Input: part model. Units: mm. Frame: model coordinates. A direction names the side the tool comes from. Round coordinates to 2 decimals unless told otherwise and drop trailing zeros. Order: outer loops, then holes, each group sorted by start corner. A loop starts at its lowest first (then second) coordinate and runs counter-clockwise, first axis right, second up. Notation, with made-up numbers: M 30.25,28 L 68.25,28 A16 ccw 68.25,55 Z; hole C 38,49.25 d7. An arc over 180 degrees is marked long. One line per question, with ' | ' between items.
```python
from build123d import *

# Parameters (mm, degrees)
SALIENTE_EXTRUIR1_DEPTH = 20
CROQUIS2_R              = 20
SALIENTE_EXTRUIR2_DEPTH = 35
CORTAR_EXTRUIR1_DEPTH   = 15
CORTAR_EXTRUIR2_REACH   = 68.332
CROQUIS4_R              = 4
CROQUIS5_R              = 12.5
CROQUIS5_R_2            = 6
SALIENTE_EXTRUIR3_DEPTH = 48
REDONDEO1_R             = 3
NERVIO1_REACH           = 91.22
CROQUIS6_WALL_W         = 207.940466532
CROQUIS6_WALL_H         = 6


with BuildPart() as part:
    # Croquis1 → Saliente-Extruir1 (new body)
    with BuildSketch(Plane.XY):
        with BuildLine():
            Line((-12.5, -26.339134382), (-12.5, -60))
            ThreePointArc((-12.5, -60), (0, -47.5), (12.5, -60))
            Line((12.5, -60), (12.5, -26.339134382))
            ThreePointArc((12.5, -26.339134382), (13.646923907, -18.12329602), (17, -10.535653753))
            ThreePointArc((17, -10.535653753), (0, -20), (-17, -10.535653753))
            ThreePointArc((-17, -10.535653753), (-13.646923907, -18.12329602), (-12.5, -26.339134382))
        make_face()
    extrude(amount=SALIENTE_EXTRUIR1_DEPTH)

    # Croquis2 → Saliente-Extruir2 (add)
    with BuildSketch(Plane.XY):
        with Locations(Location((0, 0, 0), (0, 0, 211.788330617))):
            Circle(CROQUIS2_R)
    extrude(amount=SALIENTE_EXTRUIR2_DEPTH)

    # Croquis3 → Cortar-Extruir1 (cut)
    with BuildSketch(Plane.XY.offset(35)):
        with BuildLine():
            Line((-3, 11.618950039), (-3, 8))
            Line((-3, 8), (3, 8))
            Line((3, 8), (3, 11.618950039))
            ThreePointArc((3, 11.618950039), (12, 0), (3, -11.618950039))
            Line((3, -11.618950039), (3, -8))
            Line((3, -8), (-3, -8))
            Line((-3, -8), (-3, -11.618950039))
            ThreePointArc((-3, -11.618950039), (-12, 0), (-3, 11.618950039))
        make_face()
    extrude(amount=-CORTAR_EXTRUIR1_DEPTH, mode=Mode.SUBTRACT)

    # Croquis4 → Cortar-Extruir2 (cut, up to next)
    with BuildSketch(Plane.XY.offset(20), mode=Mode.PRIVATE) as cortar_extruir2_sk1:
        Circle(CROQUIS4_R)
    cortar_extruir2_tool1 = extrude(cortar_extruir2_sk1.sketch, amount=-CORTAR_EXTRUIR2_REACH, mode=Mode.PRIVATE) & part.part
    add(cortar_extruir2_tool1.solids().sort_by_distance((0, 0, 20))[0], mode=Mode.SUBTRACT)

    # Croquis5 → Saliente-Extruir3 (add)
    with BuildSketch(Plane.XY):
        with Locations((0, -60)):
            Circle(CROQUIS5_R)
        with Locations((0, -60)):
            Circle(CROQUIS5_R_2, mode=Mode.SUBTRACT)
    extrude(amount=SALIENTE_EXTRUIR3_DEPTH)

    # Redondeo1
    redondeo1_edges = [part.edges().sort_by_distance(p)[0] for p in [
        (-12.5, -60, 48),
    ]]
    fillet(redondeo1_edges, radius=REDONDEO1_R)

    # Croquis6 wall → Nervio1 (add, up to next)
    with BuildSketch(Plane(origin=(0, -33.75, 30), x_dir=(0, -1, 0), z_dir=(0, 0, -1)), mode=Mode.PRIVATE) as nervio1_sk1:
        Rectangle(CROQUIS6_WALL_W, CROQUIS6_WALL_H)
    nervio1_tool1 = extrude(nervio1_sk1.sketch, amount=NERVIO1_REACH, mode=Mode.PRIVATE) - part.part
    add(nervio1_tool1.solids().sort_by_distance((0, -33.75, 30))[0])


solid = part.part
```
Item 1: Section query B-B, the plane y = 0. Return loops of the section in (x, z).
Report:
outline: M -20,0 L -4,0 L -4,20 L -12,20 L -12,35 L -20,35 Z; M 4,0 L 20,0 L 20,35 L 12,35 L 12,20 L 4,20 Z
Item 2: Section query D-D, the plane z = 10. Return loops of the section in (x, y).
Report:
outline: M -17,-10.54 A30 cw -12.5,-26.34 L -12.5,-60 A12.5 ccw 12.5,-60 L 12.5,-26.34 A30 cw 17,-10.54 A20 ccw long Z; hole C 0,-60 d12; hole C 0,0 d8
Item 3: Section query A-A, the plane z = 34. Return loops of the section in (x, y), plus the area to 3 significant figures.
Report:
outline: C 0,0 d40; C 0,-60 d25; hole C 0,-60 d12; hole M -3,-11.62 L -3,-8 L 3,-8 L 3,-11.62 A12 ccw 3,11.62 L 3,8 L -3,8 L -3,11.62 A12 ccw Z | area: 1,230 mm²
Item 4: Mould query, pull axis Y, two halves, no side actions, for faces 5 (the cylindrical face through (-13.68, -18.01, 9.86)), 6 (the cylindrical face through (-0.867, -3.905, 10.14)), 7 (the flat face through (-12.5, -43, 10)). Classes: +Y half, -Y half, draft (parallel to the pull), parting line (faces both ways), or undercut.
Report:
face 5: -Y half | face 6: undercut | face 7: draft
Item 5: Access query for faces 1 (the flat face through (-1, 10, 35)), 2 (the flat face through (12.5, -43, 10)), 3 (the flat face through (3, 10, 28)), 4 (the flat face through (-9, -35, 20)). Directions: +Z, -Z, +X, -X, +Y, -Y. A direction counts if a zero-diameter tool reaches every point of the face in a straight line with its end or side. Return the directions, or none.
Report:
face 1: +Z, +X, -X, +Y | face 2: +Z, -Z, +X, -Y | face 3: +Z | face 4: +Z, -X
Item 6: Line query: line 1 along Y through (x, z) = (0, 25.5); line 2 along Y through (x, z) = (0, 12); line 3 along Y through (x, z) = (0, 36). Output: solid intervals per line, ascending. Write a range as from..to.
Report:
line 1: -72.5..-66, -54..-8, 8..20 | line 2: -72.5..-66, -54..-4, 4..20 | line 3: -72.5..-66, -54..-47.5
Item 7: Section query C-C, the plane x = 0. Return loops of the section in (y, z), plus the area to 3 significant figures.
Report:
outline: M -72.5,0 L -66,0 L -66,48 L -69.5,48 A3 ccw -72.5,45 Z; M -54,0 L -4,0 L -4,20 L -8,20 L -8,35 L -20,35 L -20,30 L -47.5,30 L -47.5,45 A3 ccw -50.5,48 L -54,48 Z; M 4,0 L 20,0 L 20,35 L 8,35 L 8,20 L 4,20 Z | area: 2,450 mm²
Item 8: First-contact query: pin 1 (5 mm diameter, centred on y = -7, z = 21, fed in from -X); pin 2 (10 mm diameter, centred on y = -40.5, z = 14, fed in from +X); pin 3 (5 mm diameter, centred on x = 10, z = 28, fed in from +Y); pin 4 (7 mm diameter, centred on x = 0, y = 0, fed in from -Z). Flat tips, straight axial feed; report the tip coordinate or a pass-through.
Report:
pin 1: x = -19.49 | pin 2: x = 12.5 | pin 3: y = 18.54 | pin 4: through
